Can you work these out from the model? Positions are in its coordinate system, mm. Face numbers are marked on the shaded views. A direction names the side the tool comes from. Give positions to 0.01 mm unless a question says otherwise; leave off trailing zeros. Loops run counter-clockwise (first coordinate to the right, second up) from the corner with the lowest first, then second, coordinate; pieces in that order, holes last. Notation, with made-up numbers: M 76,6.25 L 107,6.25 A23 ccw 107,34.25 Z; hole C 47,-11 d1. An arc over 180 degrees is marked long. One line per item, written item: value. Start each with the question number.
from build123d import *

# Parameters (mm, degrees)
F1_DEPTH = 1.6
F2_W     = 3.14566
F2_H     = 3.226229
F2_R     = 0.8
F3_DEPTH = 1
F4_W     = 2.903376
F4_H     = 2.958158
F4_R     = 0.8
F5_DEPTH = 1


with BuildPart() as f1:
    # F0 (on Top) → F1 (new body)
    with BuildSketch(Plane.XY):
        Polygon((0, 3.9), (0, 0), (2.6, 0), (2.6, -4.5), (1.2, -4.5), (1.2, -10.5), (11.2, -10.5), (11.2, -4.5), (9.8, -4.5), (9.8, 0), (12.4, 0), (12.4, 3.9), (13.4, 3.9), (13.4, 5.5), (12.4, 5.5), (12.4, 9.4), (0, 9.4), (0, 5.5), (-1, 5.5), (-1, 3.9), align=None)
    extrude(amount=F1_DEPTH)

    # F2 (on face) → F3 (cut, through all)
    with BuildSketch(Plane(origin=(-1, 0, 0), x_dir=(0, -1, 0), z_dir=(-1, 0, 0))):
        with Locations((-4.643819, 0.893174)):
            Rectangle(F2_W, F2_H)
        with Locations((-4.7, 0.8)):
            Circle(F2_R, mode=Mode.SUBTRACT)
    extrude(amount=-F3_DEPTH, mode=Mode.SUBTRACT)

    # F4 (on face) → F5 (cut, through all)
    with BuildSketch(Plane.YZ.offset(13.4)):
        with Locations((4.745394, 0.737966)):
            Rectangle(F4_W, F4_H)
        with Locations((4.7, 0.8)):
            Circle(F4_R, mode=Mode.SUBTRACT)
    extrude(amount=-F5_DEPTH, mode=Mode.SUBTRACT)


solid = f1.part
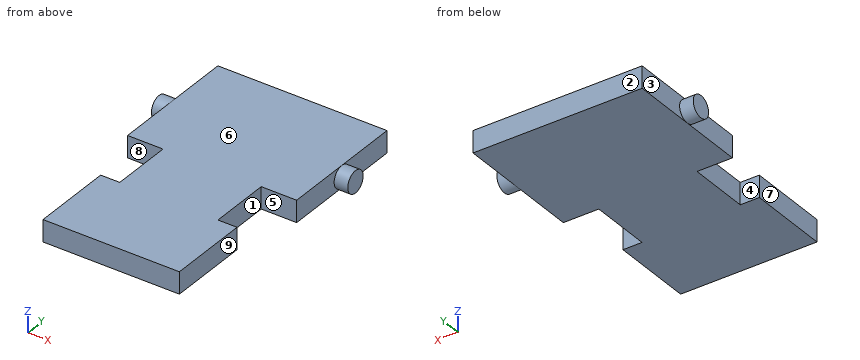
Q1. I need wall thicknesses on line 1 along Y through (x, z) = (0.5, 1.45); line 2 along X through (y, z) = (4, 1.3); line 3 along X through (y, z) = (-1, 0.45). Which ranges of each line are inside material? Lowest first, please.
Q2. If we section it at C-C, the plane y = 7.25: Write out the boundary of the cut face in (x, z).
Q3. If we mould it in two halves opening along Y, with no side actions, what happens to the marked faces 1, 2, 3 and 4? For each: released by +Y, released by -Y, zero draft, split by the parting line, or undercut.
Q4. Which directions (+Z, -Z, +X, -X, +Y, -Y) give clear straight access to the entire face, cutting with the end or side of a thin tool? Please do the marked faces 5, 6, 7, 8 and 9.
Q5. If we section it at D-D, the plane y = -2.25: Write out the boundary of the cut face in (x, z).
Q6. If we section it at A-A, the plane x = 10: Write out the boundary of the cut face in (y, z), plus the area to 3 significant figures.
Q7. For P1, Ø0.5, axis at y = -8, z = 0.5, coming from the +X side; P2, Ø0.5, axis at y = 3, z = 0.5, coming from the +X side; P3, Ø0.8, axis at y = -8.5, z = 1, coming from the -X side, each with a flat end and sliding along its axis, tell me the tip position at first contact or that it passes through.
Q8. If we section it at B-B, the plane z = 0.8: Write out the boundary of the cut face in (x, y).
Response:
1. line 1: 0 to 9.4
1. line 2: 0 to 12.4
1. line 3: 2.6 to 9.8
2. outline: M 0,0 L 12.4,0 L 12.4,1.6 L 0,1.6 Z
3. face 1: undercut
3. face 2: released by +Y
3. face 3: zero draft
3. face 4: undercut
4. face 5: +Z, -Z, +X
4. face 6: +Z, +X, -X, +Y, -Y
4. face 7: +Z, -Z, -X, -Y
4. face 8: +Z, -Z, -X
4. face 9: +Z, -Z, +X, -Y
5. outline: M 2.6,0 L 9.8,0 L 9.8,1.6 L 2.6,1.6 Z
6. outline: M -10.5,0 L -4.5,0 L -4.5,1.6 L -10.5,1.6 Z; M 0,0 L 9.4,0 L 9.4,1.6 L 0,1.6 Z
6. area: 24.6 mm^2
7. P1: x = 11.2
7. P2: x = 12.4
7. P3: x = 1.2
8. outline: M -1,3.9 L 0,3.9 L 0,0 L 2.6,0 L 2.6,-4.5 L 1.2,-4.5 L 1.2,-10.5 L 11.2,-10.5 L 11.2,-4.5 L 9.8,-4.5 L 9.8,0 L 12.4,0 L 12.4,3.9 L 13.4,3.9 L 13.4,5.5 L 12.4,5.5 L 12.4,9.4 L 0,9.4 L 0,5.5 L -1,5.5 Z
